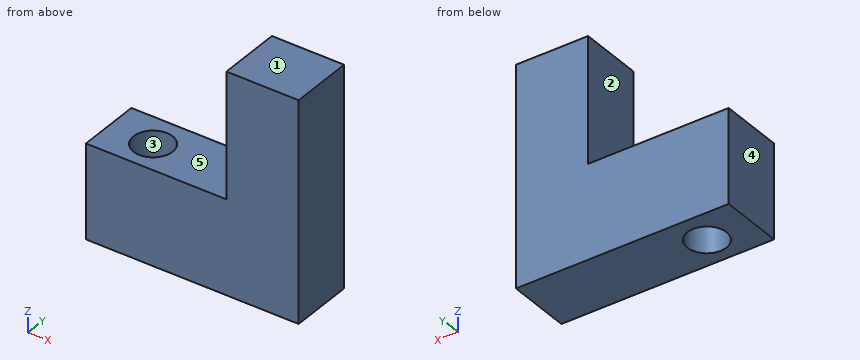
from build123d import *

# Parameters (mm, degrees)
F0_W     = 28.7874191999
F0_H     = 49.9707609415
F1_DEPTH = 25.4
F2_DEPTH = 25.4
F3_DEPTH = 25.4
F4_DEPTH = 25.4
F5_R     = 7.7956381062
F6_DEPTH = 38.1


with BuildPart() as f1:
    # F0 (on Front) → F1 (new body)
    with BuildSketch(Plane.XZ):
        with Locations((14.3937096, 24.9853804708)):
            Rectangle(F0_W, F0_H)
    extrude(amount=F1_DEPTH)

    # F0 (on Front) → F2 (join)
    with BuildSketch(Plane.XZ):
        with Locations((14.3937096, 24.9853804708)):
            Rectangle(F0_W, F0_H)
        Polygon((-56.0127794743, 0), (-56.0127794743, -37.5073552132), (28.7874191999, -37.5073552132), (28.7874191999, 0), (0, 0), align=None)
    extrude(amount=F2_DEPTH)

    # F3 (cut): a face of the model
    f3_faces = [f1.faces().sort_by_distance(p)[0] for p in [
        (0, -12.7, 24.9853804708),
    ]]
    extrude(f3_faces, amount=-F3_DEPTH, mode=Mode.SUBTRACT)

    # F0 (on Front) → F4 (join)
    with BuildSketch(Plane.XZ):
        with Locations((14.3937096, 24.9853804708)):
            Rectangle(F0_W, F0_H)
    extrude(amount=F4_DEPTH)

    # F5 (on face) → F6 (cut)
    with BuildSketch(Plane.XY):
        with Locations((-38.0956299985, -12.9956078465)):
            Circle(F5_R)
    extrude(amount=-F6_DEPTH, mode=Mode.SUBTRACT)


solid = f1.part
The listing builds one solid part. Answer for the finished solid, in the listing's coordinates (mm). Face numbers are marked on the shaded views. A direction names the side the tool comes from. Give positions to 0.01 mm unless a question says otherwise; leave off trailing zeros. Order: outer loops, then holes, each group sorted by start corner. A loop starts at its lowest first (then second) coordinate and runs counter-clockwise, first axis right, second up. Notation, with made-up numbers: (27, 0.5) - (60, 0.5) arc R21 ccw to (60, 25.5) - close; hole circle Ø3 at (6.25, -6). An arc over 180 degrees is marked (long way). One line per item, written item: value. Start each with the question number.
1) A cutting plane is placed at C-C on z = -27. Give the vertices of the cut face in (x, y), then the cut area to 3 significant figures.
2) A cutting plane is placed at A-A on x = -43. Give the vertices of the cut face in (y, z).
3) A cutting plane is placed at B-B on y = -17.25. Give the vertices of the cut face in (x, z), then the cut area to 3 significant figures.
4) The mould has two halves that part along X. Classify the marked faces 3, 4 and 5: released by +X, released by -X, zero draft, split by the parting line, or undercut.
5) A cutting plane is placed at D-D on y = -3. Give the vertices of the cut face in (x, z).
6) Given pin 1 Ø5 at (x, y) = (-4, -15) entering from +Z; pin 2 Ø12.5 at (x, y) = (-39, -12.5) entering from +Z; pin 3 Ø10 at (y, z) = (-10, 35.5) entering from -X, each flat-ended and moving along its own axis, determine where each tip first touches the part or whether it passes through.
7) Find the intervals of material crossed by L1, parallel to Z at x = -45.5, y = -4; L2, parallel to X at y = -11, z = 11, in increasing order.
8) A tool of negligible diameter and unlimited length cuts with its end or side. For the marked faces 1 and 2, from which of +Z, -Z, +X, -X, +Y, -Y can it reach the whole face along a straight path? Write none if from no direction.
Answer sheet:
1. outline: (-56.01, -25.4) - (28.79, -25.4) - (28.79, 0) - (-56.01, 0) - close; hole circle Ø15.59 at (-38.1, -13)
1. area: 1,960 mm2
2. outline: (-25.4, -37.51) - (-19.06, -37.51) - (-19.06, 0) - (-25.4, 0) - close; (-6.94, -37.51) - (0, -37.51) - (0, 0) - (-6.94, 0) - close
3. outline: (-56.01, -37.51) - (-44.63, -37.51) - (-44.63, 0) - (-56.01, 0) - close; (-31.56, -37.51) - (28.79, -37.51) - (28.79, 49.97) - (0, 49.97) - (0, 0) - (-31.56, 0) - close
3. area: 4,130 mm2
4. face 3: undercut
4. face 4: released by -X
4. face 5: zero draft
5. outline: (-56.01, -37.51) - (28.79, -37.51) - (28.79, 49.97) - (0, 49.97) - (0, 0) - (-56.01, 0) - close
6. pin 1: stops at z = 0
6. pin 2: passes through
6. pin 3: stops at x = 0
7. L1: z = -37.51 to 0
7. L2: x = 0 to 28.79
8. face 1: +Z, +X, -X, +Y, -Y
8. face 2: +Z, -X, +Y, -Y
